from build123d import *

# Parameters (mm, degrees)
SKETCH1_W           = 210
SKETCH1_H           = 112
SKETCH1_W_2         = 190
SKETCH1_H_2         = 92
BOSS_EXTRUDE1_DEPTH = 30.16
SKETCH2_W           = 210
SKETCH2_H           = 112
BOSS_EXTRUDE2_DEPTH = 4
BOSS_EXTRUDE3_DEPTH = 4.5
SKETCH5_W           = 12
SKETCH5_H           = 6
CUT_EXTRUDE2_DEPTH  = 14.5
SKETCH6_W           = 4.2
SKETCH6_H           = 3
CUT_EXTRUDE3_DEPTH  = 14.5
CHAMFER1_SIZE       = 5
CHAMFER2_SIZE       = 5
CUT_EXTRUDE4_DEPTH  = 100
FILLET1_R           = 2.1


with BuildPart() as part:
    # Sketch1 → Boss-Extrude1 (new body)
    with BuildSketch(Plane(origin=(0, 0, 0), x_dir=(1, 0, 0), z_dir=(0, 1, 0))):
        with Locations((0, 0.169761006)):
            Rectangle(SKETCH1_W, SKETCH1_H)
        Rectangle(SKETCH1_W_2, SKETCH1_H_2, mode=Mode.SUBTRACT)
    extrude(amount=BOSS_EXTRUDE1_DEPTH)

    # Sketch2 → Boss-Extrude2 (add)
    with BuildSketch(Plane.XZ):
        with Locations((0, -0.169761006)):
            Rectangle(SKETCH2_W, SKETCH2_H)
    extrude(amount=-BOSS_EXTRUDE2_DEPTH)

    # Sketch3 → Boss-Extrude3 (add)
    with BuildSketch(Plane(origin=(105, 0, 0), x_dir=(0, 0, -1), z_dir=(1, 0, 0))):
        Polygon((-42.738491713, 30.16), (43.261508287, 30.16), (36.261508287, 37.16), (-35.738491713, 37.16), align=None)
    boss_extrude3 = extrude(amount=-BOSS_EXTRUDE3_DEPTH)

    # Sketch5 → Cut-Extrude2 (cut)
    with BuildSketch(Plane.XY.offset(55.830238994)):
        with Locations((63.3, 27.16)):
            Rectangle(SKETCH5_W, SKETCH5_H)
        with Locations((17.13, 27.16)):
            Rectangle(SKETCH5_W, SKETCH5_H)
        with Locations((-29.04, 27.16)):
            Rectangle(SKETCH5_W, SKETCH5_H)
        with Locations((-75.21, 27.16)):
            Rectangle(SKETCH5_W, SKETCH5_H)
    extrude(amount=-CUT_EXTRUDE2_DEPTH, mode=Mode.SUBTRACT)

    # Sketch6 → Cut-Extrude3 (cut)
    with BuildSketch(Plane.XY.offset(55.830238994)):
        with Locations((-64.25, 28.66)):
            Rectangle(SKETCH6_W, SKETCH6_H)
        with Locations((-18.08, 28.66)):
            Rectangle(SKETCH6_W, SKETCH6_H)
        with Locations((28.09, 28.66)):
            Rectangle(SKETCH6_W, SKETCH6_H)
        with Locations((74.26, 28.66)):
            Rectangle(SKETCH6_W, SKETCH6_H)
    extrude(amount=-CUT_EXTRUDE3_DEPTH, mode=Mode.SUBTRACT)

    # Chamfer1
    chamfer1_edges = [part.edges().sort_by_distance(p)[0] for p in [
        (0, 4, -46),
        (0, 4, 46),
        (-95, 4, 0),
        (95, 4, 0),
    ]]
    chamfer(chamfer1_edges, length=CHAMFER1_SIZE)

    # Chamfer2
    chamfer2_edges = [part.edges().sort_by_distance(p)[0] for p in [
        (105, 15.08, 55.830238994),
        (-105, 15.08, 55.830238994),
        (-105, 15.08, -56.169761006),
        (105, 15.08, -56.169761006),
    ]]
    chamfer(chamfer2_edges, length=CHAMFER2_SIZE)

    # Sketch7 → Cut-Extrude4 (cut)
    with BuildSketch(Plane.XY.offset(55.830238994)):
        Polygon((100.5, 36.66), (102.75, 34.41), (102.75, 33.41), (100.5, 31.16), align=None)
    cut_extrude4 = extrude(amount=-CUT_EXTRUDE4_DEPTH, mode=Mode.SUBTRACT)

    # Mirror1: Boss-Extrude3, Cut-Extrude4 across plane
    add(boss_extrude3.mirror(Plane(origin=(0, 0, 0), x_dir=(0, 0, 1), z_dir=(1, 0, 0))))
    add(cut_extrude4.mirror(Plane(origin=(0, 0, 0), x_dir=(0, 0, 1), z_dir=(1, 0, 0))), mode=Mode.SUBTRACT)

    # Fillet1
    fillet1_edges = [part.edges().sort_by_distance(p)[0] for p in [
        (76.36, 27.16, 50.915119497),
        (30.19, 27.16, 50.915119497),
        (-15.98, 27.16, 50.915119497),
        (-62.15, 27.16, 50.915119497),
        (72.16, 27.16, 50.915119497),
        (25.99, 27.16, 50.915119497),
        (-20.18, 27.16, 50.915119497),
        (-66.35, 27.16, 50.915119497),
    ]]
    fillet(fillet1_edges, radius=FILLET1_R - 0.0001)  # a hair under: the kernel refuses the full size


solid = part.part
Here's how the part is built. I have some questions about the finished solid (model axes, mm). A direction names the side the tool comes from. Round coordinates to 2 decimals unless told otherwise and drop trailing zeros. Loops run counter-clockwise (first coordinate to the right, second up) from the corner with the lowest first, then second, coordinate; pieces in that order, holes last. Notation, with made-up numbers: (45, 76) - (58, 76) arc R21 cw to (58, 103) - close; hole circle Ø11 at (-38, 42.25). An arc over 180 degrees is marked (long way). One line per question, with ' | ' between items. Start each with the question number.
Q1. Please list where these lines run through material, in increasing order: line 1 (Z direction, x = 9, y = 17.5); line 2 (X direction, y = 15, z = 43); line 3 (Y direction, x = -96, z = 25). Write a range as [from, to].
Q2. Will these pins go through, and if not, where does the flat tip stop? pin 1 (8 mm diameter, centred on x = -29, z = 50, fed in from +Y); pin 2 (2.5 mm diameter, centred on x = -67, z = 49, fed in from +Y); pin 3 (2 mm diameter, centred on x = -1.5, z = -18.5, fed in from +Y).
Q3. I want a section at D-D (x = -84). Write out the boundary of the cut face in (y, z), then the cut area to 3 significant figures.
Q4. I want a section at A-A (y = 15.5). Write out the boundary of the cut face in (x, z), then the cut area to 3 significant figures.
Q5. We'd pull the mould along X, two halves only. Please class faces 1 (the flat face through (103.28, 33.61, -39.81)), 2 (the flat face through (102.46, 14.87, 53.37)), 3 (the flat face through (-69.21, 27, 51)), 4 (the flat face through (-105, 18, 1)): +X half, -X half, draft (parallel to the pull), parting line (faces both ways), or undercut.
Q6. I want a section at C-C (x = -26). Write out the boundary of the cut face in (y, z), then the cut area to 3 significant figures.
Q7. I want a section at B-B (z = -24). Write out the boundary of the cut face in (x, y), then the cut area to 3 significant figures.
Q8. For faces 5 (the flat face through (-1, 19, -46)), 6 (the flat face through (-1, 0, -1)), 7 (the flat face through (11.13, 27, 51)), which set-ups out of +Z, -Z, +X, -X, +Y, -Y let a thin tool reach every point of the face, with its end or its side?
Response values:
1) line 1: z = [-56.17, -46], [46, 55.83] | line 2: x = [-105, -95], [95, 105] | line 3: y = [0, 30.16]
2) pin 1: stops at y = 24.16 | pin 2: stops at y = 30.16 | pin 3: stops at y = 4
3) outline: (0, -56.17) - (30.16, -56.17) - (30.16, -46) - (9, -46) - (4, -41) - (4, 41) - (9, 46) - (30.16, 46) - (30.16, 55.83) - (0, 55.83) - close | area: 996 mm²
4) outline: (-105, -51.17) - (-100, -56.17) - (100, -56.17) - (105, -51.17) - (105, 50.83) - (100, 55.83) - (-100, 55.83) - (-105, 50.83) - close; hole (-95, -46) - (95, -46) - (95, 46) - (-95, 46) - close | area: 5,990 mm²
5) face 1: draft | face 2: +X half | face 3: undercut | face 4: -X half
6) outline: (0, -56.17) - (30.16, -56.17) - (30.16, -46) - (9, -46) - (4, -41) - (4, 41) - (9, 46) - (24.16, 46) - (24.16, 55.83) - (0, 55.83) - close | area: 937 mm²
7) outline: (-105, 0) - (105, 0) - (105, 37.16) - (100.5, 37.16) - (100.5, 36.66) - (102.75, 34.41) - (102.75, 33.41) - (100.5, 31.16) - (100.5, 30.16) - (95, 30.16) - (95, 9) - (90, 4) - (-90, 4) - (-95, 9) - (-95, 30.16) - (-100.5, 30.16) - (-100.5, 31.16) - (-102.75, 33.41) - (-102.75, 34.41) - (-100.5, 36.66) - (-100.5, 37.16) - (-105, 37.16) - close | area: 1,440 mm²
8) face 5: +Y | face 6: +Z, -Z, +X, -X, -Y | face 7: +Z, +Y
